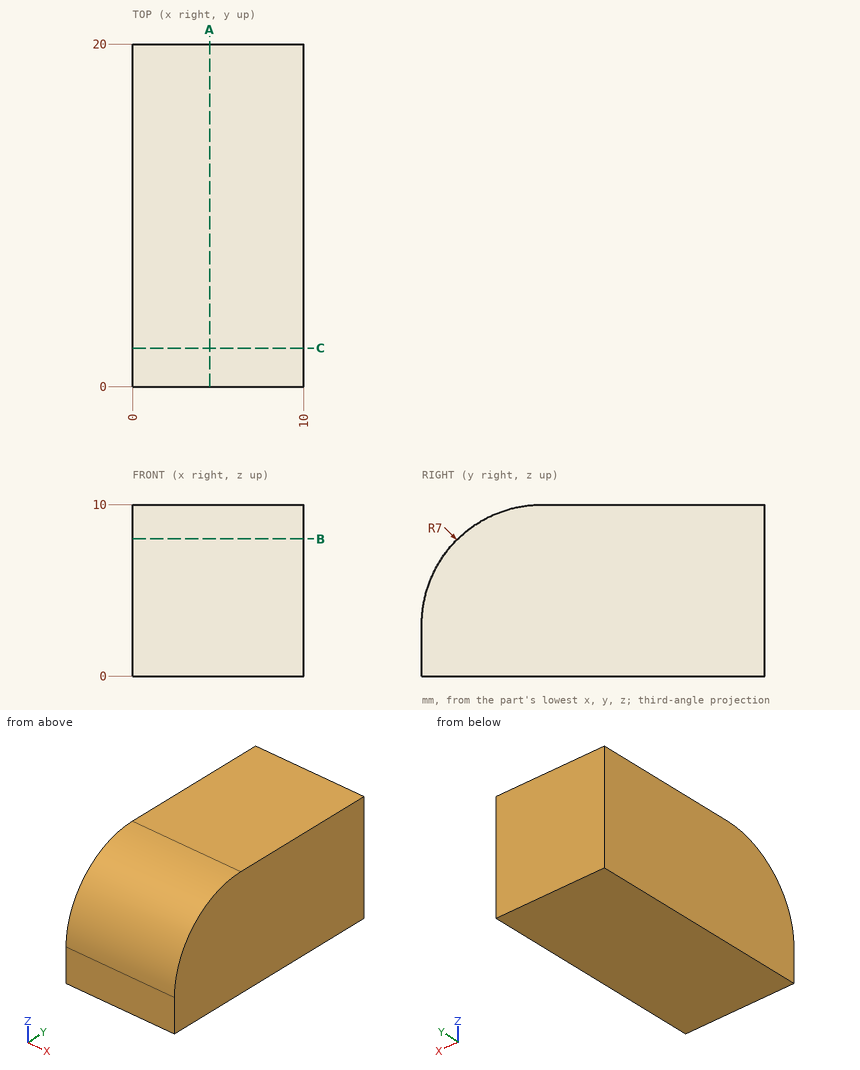
Study the drawing (mm; zero at the part's minimum x, y, z) and answer. Give positions to 0.01 mm unless a question says otherwise; leave off trailing zeros. Write each loop counter-clockwise with the first axis right and the second up, starting at its lowest first coordinate (ties: lowest second). Pieces come first, ordered by that corner, then holes. Notation, with made-up numbers: M 46,84 L 57,84 A22 ccw 57,99 Z; hole C 37,25 d2. An arc over 180 degrees is marked long. Put each result on its own line as item: value. Start each with the question number.
1. Consider line 1 along Y through (x, z) = (3.5, 4); line 2 along Z through (x, y) = (7.75, 2.5); line 3 along Z through (x, y) = (8.25, 5.75). Determine where each line is inside the solid, lowest interval first.
2. The part is cut by section A-A, the plane x = 4.5. Give the vertices of the cut face in (y, z), and give its area (3 significant figures).
3. The part is cut by section C-C, the plane y = 2.25. Give the vertices of the cut face in (x, z).
4. The part is cut by section B-B, the plane z = 8. Give the vertices of the cut face in (x, y), and give its area (3 significant figures).
Final values:
1. line 1: y = 0.07 to 20
1. line 2: z = 0 to 8.36
1. line 3: z = 0 to 9.89
2. outline: M 0,0 L 20,0 L 20,10 L 7,10 A7 ccw 0,3 Z
2. area: 189 mm²
3. outline: M 0,0 L 10,0 L 10,8.14 L 0,8.14 Z
4. outline: M 0,2.1 L 10,2.1 L 10,20 L 0,20 Z
4. area: 179 mm²
